Check sheet for the modelled part. Datum: model origin and axes. Units: mm. A direction names the side the tool comes from. Round coordinates to 2 decimals unless told otherwise and drop trailing zeros. Write each loop counter-clockwise with the first axis right and the second up, starting at its lowest first coordinate (ties: lowest second). Pieces come first, ordered by that corner, then holes. Notation, with made-up numbers: (-5.5, 33.25) - (45.5, 33.25) arc R29 cw to (45.5, 56.25) - close; hole circle Ø10 at (88.25, 4). An arc over 180 degrees is marked (long way). Answer as a JSON object with one key per item and string values. Group by question number.
Item 1: Sectioned sample at A-A on y = 0. Record the boundary of the cut face in (x, z).
Item 2: Gauge pin test, flat ends, axial feed: P1, Ø1.3, axis at x = 1, z = 11, coming from the -Y side; P2, Ø0.6, axis at x = 1, z = 11, coming from the +Y side; P3, Ø0.6, axis at x = -0.5, z = 10.5, coming from the -Y side. Record the tip position at first contact, or that the pin passes through.
Item 3: Thickness scan on line 1 (Z direction, x = -1.25, y = 2.75); line 2 (X direction, y = 1.5, z = 9.25); line 3 (X direction, y = -2.75, z = 4.5). Record the ranges inside material, lowest first.
Item 4: Release check for a two-part mould opening along Y. For faces 4 (the flat face through (0, 0, 11.65)), 5 (the cylindrical face through (-0.1, 3.9, 9.2)), 6 (the flat face through (1, 2.45, 11)) record: pulls with the +Y half, pulls with the -Y half, needs draft (parallel to the pull), parting line crosses it, or undercut.
Item 5: Set-up check for faces 1 (the cylindrical face through (0.1, -3.9, 9.2)), 2 (the flat face through (1, 2.75, 11)), 3 (the flat face through (-1, -2.45, 11)): record each of +Z, -Z, +X, -X, +Y, -Y from which the full face is reachable in a straight line by a thin tool's end or side.
Item 6: Sectioned sample at B-B on z = 1.25. Record the boundary of the cut face in (x, y), plus the area to 3 significant figures.
Autodesk Inventor part; units mm, degrees
ref_plane "YZ Plane" through (0, 0, 0) normal (1, 0, 0) x (0, 1, 0)
ref_plane "XZ Plane" through (0, 0, 0) normal (0, 1, 0) x (-1, 0, 0)
ref_plane "XY Plane" through (0, 0, 0) normal (0, 0, 1) x (1, 0, 0)
sketch "Sketch1" plane through (0, 0, 0) normal (0, 0, 1) x (1, 0, 0)
  point P0 (0, 0)
sketch "Sketch2" plane through (0, 0, 0) normal (0, 0, 1) x (1, 0, 0)
  line L0 (-3.3, 2.2605) -> (-3.3, -2.2605)
  line L1 (3.3, 2.2605) -> (3.3, -2.2605)
  arc A0 (-3.3, -2.2605) -> (3.3, -2.2605) centre (0, 0) ccw
  arc A1 (3.3, 2.2605) -> (-3.3, 2.2605) centre (0, 0) ccw
  dimension "d1" = 6.6
  dimension "d2" = 4
extrude "Extrusion1" add sketch "Sketch2" along normal blind 9
sketch "Sketch3" plane through (0, 0, 9) normal (0, 0, 1) x (1, 0, 0)
  point P0 (0, 0)
sketch "Sketch4" plane through (0, 0, 9) normal (0, 0, 1) x (1, 0, 0)
  line L0 (-3.3, 2.2605) -> (-3.3, -2.2605)
  arc A0 (-3.3, -2.2605) -> (3.3, -2.2605) centre (0, 0) ccw
  line L1 (3.3, -2.2605) -> (3.3, 2.2605)
  arc A1 (3.3, 2.2605) -> (-3.3, 2.2605) centre (0, 0) ccw
  line L2 (-3.2, 2.2293) -> (-3.2, -2.2293)
  arc A2 (-3.2, -2.2293) -> (3.2, -2.2293) centre (0, 0) ccw
  line L3 (3.2, -2.2293) -> (3.2, 2.2293)
  arc A3 (3.2, 2.2293) -> (-3.2, 2.2293) centre (0, 0) ccw
  dimension "d5" = 0.1
extrude "Extrusion2" add sketch "Sketch4" along normal blind 1 contours A3 L3 A2 L2
fillet "Fillet1" radius 0.5 4 edges at (3.2, 0, 10) (0, 3.9, 10) (-3.2, 0, 10) (0, -3.9, 10)
sketch "Sketch5" plane through (0, 0, 10) normal (0, 0, 1) x (1, 0, 0)
  circle A0 centre (0, 0) radius 1.75
  dimension "d9" = 3.5
extrude "Extrusion3" add sketch "Sketch5" along normal blind 1.65
fillet "Fillet2" radius 0.5 1 edges at (-1.75, 0, 11.65)
sketch "Sketch6" plane through (0, 0, 10) normal (0, 0, 1) x (1, 0, 0)
  circle A0 centre (0, 0) radius 1.75
  line L0 (0, -2.75) -> (-1.2, -2.75)
  line L1 (-1.2, -2.75) -> (-1.2, -2.45)
  line L2 (-1.2, -2.45) -> (0, -2.45)
  line L3 (0, -2.45) -> (0, -2.75)
  line L4 (0, 2.45) -> (1.2, 2.45)
  line L5 (1.2, 2.45) -> (1.2, 2.75)
  line L6 (1.2, 2.75) -> (0, 2.75)
  line L7 (0, 2.75) -> (0, 2.45)
  point P0 (1.4682, 1.2)
  dimension "d21" = 1.2
  dimension "d22" = 0.3
  dimension "d23" = 1.2
  dimension "d24" = 0.3
  dimension "d25" = 0.7
  dimension "d26" = 0.7
extrude "Extrusion4" add sketch "Sketch6" along normal blind 1.65 contours L0 L1 L2 L3 | L7 L6 L5 L4
properties part number "J024 motor"
Completed:
{
 "1": {"outline": "(-3.3, 0) - (3.3, 0) - (3.3, 9) - (3.2, 9) - (3.2, 9.5) arc R0.5 ccw to (2.7, 10) - (1.75, 10) - (1.75, 11.15) arc R0.5 ccw to (1.25, 11.65) - (-1.25, 11.65) arc R0.5 ccw to (-1.75, 11.15) - (-1.75, 10) - (-2.7, 10) arc R0.5 ccw to (-3.2, 9.5) - (-3.2, 9) - (-3.3, 9) - close"},
 "2": {"P1": "y = -1.71", "P2": "y = 2.75", "P3": "y = -2.75"},
 "3": {"line 1": "0 to 10", "line 2": "-3.2 to 3.2", "line 3": "-2.9 to 2.9"},
 "4": {"face 4": "needs draft", "face 5": "pulls with the +Y half", "face 6": "undercut"},
 "5": {"face 1": "+Z, -Y", "face 2": "+Z, +X, -X, +Y", "face 3": "+Z, +X, -X"},
 "6": {"outline": "(-3.3, -2.26) arc R4 ccw to (3.3, -2.26) - (3.3, 2.26) arc R4 ccw to (-3.3, 2.26) - close", "area": "46.0 mm²"}
}
